from build123d import *

# Parameters (mm, degrees)
ESBO_O1_R                = 10.75
RESSALTO_EXTRUS_O1_DEPTH = 4
ESBO_O2_R                = 3
RESSALTO_EXTRUS_O2_DEPTH = 13.7
FILETE2_R                = 1
ESBO_O3_R                = 0.5
CORTE_EXTRUS_O1_DEPTH    = 21.464970071


with BuildPart() as part:
    # Esboço1 → Ressalto-extrusão1 (new body)
    with BuildSketch(Plane.XY):
        Circle(ESBO_O1_R)
    extrude(amount=RESSALTO_EXTRUS_O1_DEPTH)

    # Esboço2 → Ressalto-extrusão2 (add)
    with BuildSketch(Plane.XY.offset(4)):
        with Locations(Location((0, 0, 0), (0, 0, 180))):
            Circle(ESBO_O2_R)
    extrude(amount=RESSALTO_EXTRUS_O2_DEPTH)

    # Filete2
    filete2_edges = [part.edges().sort_by_distance(p)[0] for p in [
        (3, 0, 4),
    ]]
    fillet(filete2_edges, radius=FILETE2_R)

    # Esboço3 → Corte-extrusão1 (cut, through all)
    with BuildSketch(Plane.XY.offset(4)):
        with Locations((7.1, 0)):
            Circle(ESBO_O3_R)
        with Locations((-7.1, 0)):
            Circle(ESBO_O3_R)
        with Locations((0, 7.1)):
            Circle(ESBO_O3_R)
        with Locations((0, -7.1)):
            Circle(ESBO_O3_R)
    extrude(amount=-CORTE_EXTRUS_O1_DEPTH, mode=Mode.SUBTRACT)


solid = part.part
Verification items for the finished model (mm, model axes). A direction names the side the tool comes from. Coordinates: 2 decimals unless noted, no trailing zeros. Order: outer loops, then holes, each group sorted by start corner. A loop starts at its lowest first (then second) coordinate and runs counter-clockwise, first axis right, second up.
Item 1: Depth check by flat-ended pin: pin 1 (5 mm diameter, centred on y = -2, z = 2, fed in from +X); pin 2 (10 mm diameter, centred on y = -4, z = 8.5, fed in from +X); pin 3 (4 mm diameter, centred on x = -4.5, z = 12.5, fed in from +Y); pin 4 (1 mm diameter, centred on y = -4, z = 7.5, fed in from -X). Enter the tip coordinate at first touch or a pass-through.
Filled in:
pin 1: stops at x = 10.75
pin 2: stops at x = 10.59
pin 3: stops at y = 1.66
pin 4: passes through
Item 2: Release check for a two-part mould opening along X. For faces 1 (the face through (0, 0, 0)), 2 (the face through (-1.4, 10.66, 1.97)), 3 (the face through (-6.623, 0.15, 2.028)) record: +X half, -X half, draft (parallel to the pull), parting line (faces both ways), or undercut.
Filled in:
face 1: draft
face 2: parting line
face 3: undercut
Item 3: Section check A-A, the plane x = 0. Enter the section's corners in (y, z), then the cut area to 3 significant figures.
Filled in:
outline: (-10.75, 0) - (-7.6, 0) - (-7.6, 4) - (-10.75, 4) - close; (-6.6, 0) - (6.6, 0) - (6.6, 4) - (4, 4) arc R1 cw to (3, 5) - (3, 17.7) - (-3, 17.7) - (-3, 5) arc R1 cw to (-4, 4) - (-6.6, 4) - close; (7.6, 0) - (10.75, 0) - (10.75, 4) - (7.6, 4) - close
area: 161 mm2
Item 4: Section check B-B, the plane z = 3. Enter the section's corners in (x, y), then the cut area to 3 significant figures.
Filled in:
outline: circle Ø21.5 at (0, 0); hole circle Ø1 at (-7.1, 0); hole circle Ø1 at (0, -7.1); hole circle Ø1 at (0, 7.1); hole circle Ø1 at (7.1, 0)
area: 360 mm2
Item 5: Material ranges on L1, parallel to Y at x = 0, z = 2.8; L2, parallel to Z at x = 5.25, y = 8; L3, parallel to Y at x = -7.1, z = 1.15, recorded low to high.
Filled in:
L1: y = -10.75 to -7.6, -6.6 to 6.6, 7.6 to 10.75
L2: z = 0 to 4
L3: y = -8.07 to -0.5, 0.5 to 8.07
Item 6: Section check C-C, the plane y = 7.1. Enter the section's corners in (x, z), then the cut area to 3 significant figures.
Filled in:
outline: (-8.07, 0) - (-0.5, 0) - (-0.5, 4) - (-8.07, 4) - close; (0.5, 0) - (8.07, 0) - (8.07, 4) - (0.5, 4) - close
area: 60.6 mm2
Item 7: Access from +Z, -Z, +X, -X, +Y, -Y to the whole of each face (thin tool, end or side, straight path). Record for faces 4 (the face through (-2.86, -0.9, 11.26)), 5 (the face through (0, 0, 17.7)).
Filled in:
face 4: +Z
face 5: +Z, +X, -X, +Y, -Y
